Design review of the part built by this model. Coordinates are the model's own, in mm. A direction names the side the tool comes from. Give positions to 0.01 mm unless a question says otherwise; leave off trailing zeros. Loops run counter-clockwise (first coordinate to the right, second up) from the corner with the lowest first, then second, coordinate; pieces in that order, holes last. Notation, with made-up numbers: M -8,39.25 L 9,39.25 A22 cw 9,69.25 Z; hole C -38,-2 d10. An arc over 180 degrees is marked long. Answer as CSV lines item,"result".
```python
from build123d import *

# Parameters (mm, degrees)
SKETCH1_W           = 87
SKETCH1_H           = 50.8
BOSS_EXTRUDE1_DEPTH = 33.8
BOSS_EXTRUDE2_DEPTH = 2
SKETCH5_R           = 13.034233904
BOSS_EXTRUDE4_DEPTH = 10


with BuildPart() as part:
    # Sketch1 → Boss-Extrude1 (new body)
    with BuildSketch(Plane(origin=(0, 0, 0), x_dir=(1, 0, 0), z_dir=(0, 1, 0))):
        with Locations((43.5, 25.4)):
            Rectangle(SKETCH1_W, SKETCH1_H)
    extrude(amount=BOSS_EXTRUDE1_DEPTH)

    # Sketch2 → Boss-Extrude2 (add)
    with BuildSketch(Plane.XZ):
        with BuildLine():
            Line((0, -42.9), (-10.5, -42.9))
            Line((-10.5, -42.9), (-10.5, -27.4))
            Line((-10.5, -27.4), (-6.5, -27.4))
            ThreePointArc((-6.5, -27.4), (-4.5, -25.4), (-6.5, -23.4))
            Line((-6.5, -23.4), (-10.5, -23.4))
            Line((-10.5, -23.4), (-10.5, -7.9))
            Line((-10.5, -7.9), (0, -7.9))
            Line((0, -7.9), (0, -42.9))
        make_face()
        with BuildLine():
            Line((97.5, -23.4), (97.5, -7.9))
            Line((97.5, -7.9), (87, -7.9))
            Line((87, -7.9), (87, -42.9))
            Line((87, -42.9), (97.5, -42.9))
            Line((97.5, -42.9), (97.5, -27.4))
            Line((97.5, -27.4), (93.5, -27.4))
            ThreePointArc((93.5, -27.4), (91.5, -25.4), (93.5, -23.4))
            Line((93.5, -23.4), (97.5, -23.4))
        make_face()
    extrude(amount=-BOSS_EXTRUDE2_DEPTH)

    # Sketch5 → Boss-Extrude4 (add)
    with BuildSketch(Plane(origin=(87, 0, 0), x_dir=(0, 0, -1), z_dir=(1, 0, 0))):
        with Locations((25.146357233, 17.068762313)):
            Circle(SKETCH5_R)
    extrude(amount=BOSS_EXTRUDE4_DEPTH)


solid = part.part
```
1. We need section A-A, the plane z = -25.4. Write out the cut boundary in (x, y), plus the area to 3 significant figures.
Answer block:
outline,"M -4.5,0 L 91.5,0 L 91.5,2 L 87,2 L 87,4.04 L 97,4.04 L 97,30.1 L 87,30.1 L 87,33.8 L 0,33.8 L 0,2 L -4.5,2 Z"
area,"3,220 mm²"
2. We need section C-C, the plane z = -20. Write out the cut boundary in (x, y).
Answer block:
outline,"M -10.5,0 L 97.5,0 L 97.5,2 L 87,2 L 87,5.09 L 97,5.09 L 97,29.04 L 87,29.04 L 87,33.8 L 0,33.8 L 0,2 L -10.5,2 Z"
3. For faces 1 (the cylindrical face through (91.5, 1, -25.4)), 2 (the flat face through (97, 17, -25)), 3 (the flat face through (-4, 2, -25)), list the 3-axis set-ups (+Z, -Z, +X, -X, +Y, -Y) from which the entire face can be reached by the end or side of a thin tool; tool diameter is ignored.
Answer block:
face 1,"+X, -Y"
face 2,"+Z, -Z, +X, +Y"
face 3,"+Z, -Z, -X, +Y"
4. To check wall thickness, follow L1, parallel to X at y = 17, z = -33; L2, parallel to X at y = 9, z = -39.5; L3, parallel to Y at x = -2, z = -31. State the ranges of each line that lie inside material, in increasing order. Write a range as [from, to].
Answer block:
L1,"[0, 97]"
L2,"[0, 87]"
L3,"[0, 2]"
5. We need section B-B, the plane y = 19.5. Write out the cut boundary in (x, z), plus the area to 3 significant figures.
Answer block:
outline,"M 0,-50.8 L 87,-50.8 L 87,-37.95 L 97,-37.95 L 97,-12.34 L 87,-12.34 L 87,0 L 0,0 Z"
area,"4,680 mm²"
6. We need section D-D, the plane y = 12. Write out the cut boundary in (x, z).
Answer block:
outline,"M 0,-50.8 L 87,-50.8 L 87,-37.15 L 97,-37.15 L 97,-13.14 L 87,-13.14 L 87,0 L 0,0 Z"
7. The part is to be moulded in two halves that separate along Z. For faces 4 (the flat face through (43, 33.8, -26)), 5 (the flat face through (-5, 1, -7.9)), 6 (the flat face through (95, 1, -23.4)), say which applies: pulls with the +Z half, pulls with the -Z half, needs draft (parallel to the pull), parting line crosses it, or undercut.
Answer block:
face 4,"needs draft"
face 5,"pulls with the +Z half"
face 6,"undercut"
8. For P1, Ø8.5, axis at x = 92.5, z = -24.5, coming from the +Y side; P2, Ø10, axis at y = 22.5, z = -11, coming from the -X side; P3, Ø1, axis at x = 95.5, y = 0.5, coming from the -Z side, all flat-tipped, find the tip position at first contact; note any pin that passes through.
Answer block:
P1,"y = 30.1"
P2,"x = 0"
P3,"z = -42.9"
